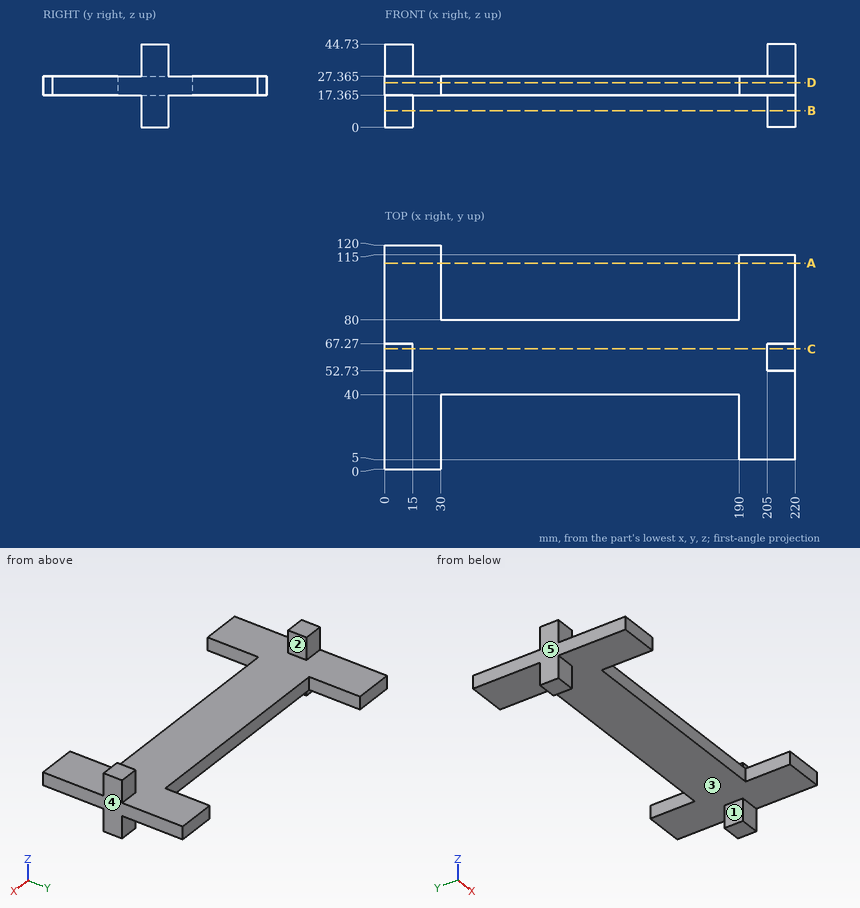
Geometry: see drawing. Coordinates: mm, zero at the bounding-box minimum. A direction names the side the tool comes from. Round coordinates to 2 decimals unless told otherwise and drop trailing zeros. Order: outer loops, then holes, each group sorted by start corner. A loop starts at its lowest first (then second) coordinate and runs counter-clockwise, first axis right, second up. Notation, with made-up numbers: (67.25, 80.25) -> (105.25, 80.25) arc R16 ccw to (105.25, 86.25) -> close; hole circle Ø11 at (-30, -31.5). An arc over 180 degrees is marked (long way). Use CSV: the item, a comma, the result in double quotes.
(1) Section B-B on z = 9. Return the cut outline in (x, y).
Report:
outline,"(0, 52.73) -> (15, 52.73) -> (15, 67.27) -> (0, 67.27) -> close; (205, 52.73) -> (220, 52.73) -> (220, 67.27) -> (205, 67.27) -> close"
(2) Section C-C on y = 64.5. Return the cut outline in (x, z) (3 decimals).
Report:
outline,"(0, 0) -> (15, 0) -> (15, 17.365) -> (205, 17.365) -> (205, 0) -> (220, 0) -> (220, 44.73) -> (205, 44.73) -> (205, 27.365) -> (15, 27.365) -> (15, 44.73) -> (0, 44.73) -> close"
(3) Section A-A on y = 110.5. Return the cut outline in (x, z) (3 decimals).
Report:
outline,"(0, 17.365) -> (30, 17.365) -> (30, 27.365) -> (0, 27.365) -> close; (190, 17.365) -> (220, 17.365) -> (220, 27.365) -> (190, 27.365) -> close"
(4) First-contact query: pin 1 Ø4.5 at (x, z) = (8.5, 36) entering from +Y; pin 2 Ø8 at (x, z) = (141.5, 27.5) entering from -Y; pin 3 Ø8 at (x, z) = (200.5, 20) entering from +Y. Flat tips, straight axial feed; report the tip coordinate or a pass-through.
Report:
pin 1,"y = 67.27"
pin 2,"y = 40"
pin 3,"y = 115"
(5) Access query for the marked faces 1 and 2. Directions: +Z, -Z, +X, -X, +Y, -Y. A direction counts if a zero-diameter tool reaches every point of the face in a straight line with its end or side. Return the directions, or none.
Report:
face 1,"-Z, +Y, -Y"
face 2,"+Z, +Y, -Y"
(6) Pull-direction query (X, two-part tool) for the marked faces 3, 4 and 5; classes: +X half, -X half, draft (parallel to the pull), parting line (faces both ways), or undercut.
Report:
face 3,"undercut"
face 4,"+X half"
face 5,"-X half"
(7) Section D-D on z = 24. Return the cut outline in (x, y).
Report:
outline,"(0, 0) -> (30, 0) -> (30, 40) -> (190, 40) -> (190, 5) -> (220, 5) -> (220, 115) -> (190, 115) -> (190, 80) -> (30, 80) -> (30, 120) -> (0, 120) -> close"
(8) Ray query, L1, parallel to X at y = 107.5, z = 18; L2, parallel to X at y = 67, z = 5.5; L3, parallel to Z at x = 193, y = 53.5 (3 decimals). Return the intervals inside material, ascending.
Report:
L1,"0 to 30, 190 to 220"
L2,"0 to 15, 205 to 220"
L3,"17.365 to 27.365"
